Input: dimensioned drawing with shaded views. Units: mm. Origin: part minimum x, y, z. A direction names the side the tool comes from. Coordinates: 2 decimals unless noted, no trailing zeros. Write each loop counter-clockwise with the first axis right and the second up, starting at its lowest first coordinate (ties: lowest second). Pieces come first, ordered by that corner, then holes. Notation, with made-up numbers: M 82.5,39.5 L 107.5,39.5 A8 cw 107.5,51.5 Z; hole C 45,66 d9. An arc over 180 degrees is marked long. Use one line per item in the form item = value.
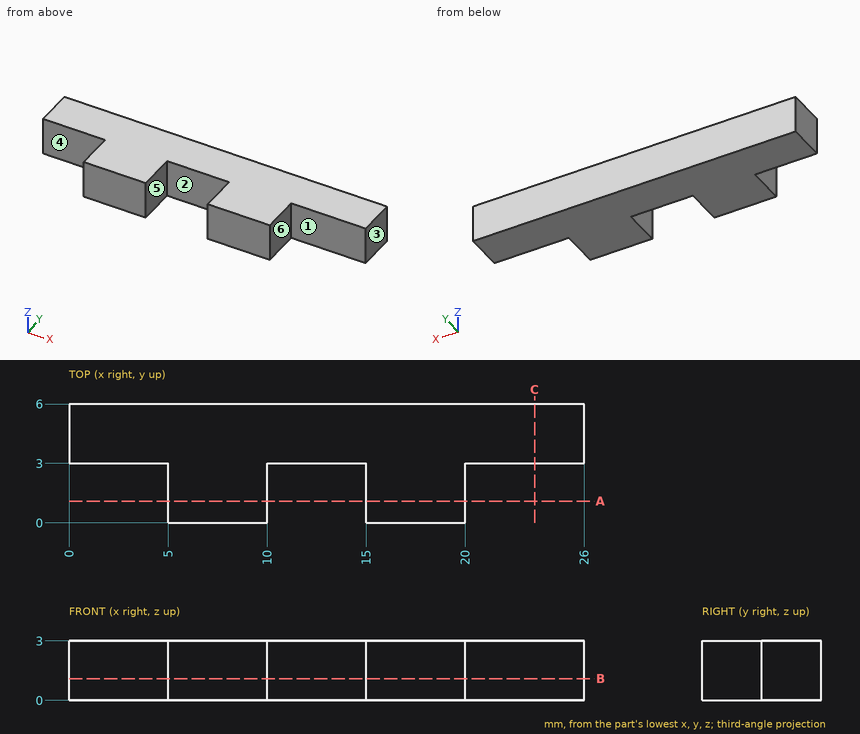
(1) Section query A-A on y = 1.1. Return the cut outline in (x, z), plus the area to 3 significant figures.
Computed:
outline = M 5,0 L 10,0 L 10,3 L 5,3 Z; M 15,0 L 20,0 L 20,3 L 15,3 Z
area = 30.0 mm^2
(2) Section query B-B on z = 1.1. Return the cut outline in (x, y), plus the area to 3 significant figures.
Computed:
outline = M 0,3 L 5,3 L 5,0 L 10,0 L 10,3 L 15,3 L 15,0 L 20,0 L 20,3 L 26,3 L 26,6 L 0,6 Z
area = 108 mm^2
(3) Section query C-C on x = 23.5. Return the cut outline in (y, z).
Computed:
outline = M 3,0 L 6,0 L 6,3 L 3,3 Z
(4) Line query: probe 1 along X at (y, z) = (2.05, 0.4); probe 2 along Y at (x, z) = (13, 1.6). Output: solid intervals per line, ascending.
Computed:
probe_1 = 5 to 10, 15 to 20
probe_2 = 3 to 6
(5) Pull-direction query (X, two-part tool) for the marked faces 1, 2 and 3; classes: pulls with the +X half, pulls with the -X half, needs draft (parallel to the pull), parting line crosses it, or undercut.
Computed:
face_1 = needs draft
face_2 = undercut
face_3 = pulls with the +X half
(6) Set-up query: the marked faces 4, 5 and 6. Return all of +Z, -Z, +X, -X, +Y, -Y with unobstructed straight access to the full face (end or side cutting, diameter ignored); none if empty.
Computed:
face_4 = +Z, -Z, -X, -Y
face_5 = +Z, -Z, -Y
face_6 = +Z, -Z, +X, -Y
(7) First-contact query: pin 1 Ø1.5 at (x, z) = (2.5, 1.5) entering from -Y; pin 2 Ø0.9 at (y, z) = (1, 2) entering from -X; pin 3 Ø0.9 at (y, z) = (1, 2) entering from +X. Flat tips, straight axial feed; report the tip coordinate or a pass-through.
Computed:
pin_1 = 3
pin_2 = 5
pin_3 = 20
